Here's how the part is built. I have some questions about the finished solid (model axes, mm). Face numbers are marked on the shaded views. Coordinates: 2 decimals unless noted, no trailing zeros. Write each loop counter-clockwise with the first axis right and the second up, starting at its lowest first coordinate (ties: lowest second). Pieces come first, ordered by that corner, then holes. Notation, with made-up numbers: M -7.5,35 L 31.5,35 A20 cw 31.5,46 Z; hole C 65,51.25 d2. An arc over 180 degrees is marked long. Use a Markdown table: item, result.
```python
from build123d import *

# Parameters (mm, degrees)
CROQUIS1_R              = 5
CROQUIS1_R_2            = 4.05
SALIENTE_EXTRUIR1_DEPTH = 3
CROQUIS5_W              = 3
CROQUIS5_H              = 21
SALIENTE_EXTRUIR3_DEPTH = 8
CROQUIS11_W             = 3
CROQUIS11_H             = 21
SALIENTE_EXTRUIR6_DEPTH = 8
CORTAR_EXTRUIR3_DEPTH   = 34
CORTAR_EXTRUIR4_DEPTH   = 3
SALIENTE_EXTRUIR8_DEPTH = 8
CROQUIS15_R             = 1.55
CORTAR_EXTRUIR6_DEPTH   = 7
CROQUIS16_R             = 2.8
CROQUIS16_R_2           = 1.55
CORTAR_EXTRUIR7_DEPTH   = 3


with BuildPart() as part:
    # Croquis1 → Saliente-Extruir1 (new body)
    with BuildSketch(Plane(origin=(0, 0, 0), x_dir=(1, 0, 0), z_dir=(0, 1, 0))):
        Polygon((0, 32), (25.301087099, 32), (25.301087099, -7), (19.301087099, -13), (-1.698912901, -13), (-7.698912901, -7), (-7.698912901, 32), align=None)
        Circle(CROQUIS1_R, mode=Mode.SUBTRACT)
        with Locations((17, 0)):
            Circle(CROQUIS1_R_2, mode=Mode.SUBTRACT)
    extrude(amount=SALIENTE_EXTRUIR1_DEPTH)

    # Croquis5 → Saliente-Extruir3 (add)
    with BuildSketch(Plane.XZ):
        with Locations((-6.198912901, -18.5)):
            Rectangle(CROQUIS5_W, CROQUIS5_H)
    extrude(amount=SALIENTE_EXTRUIR3_DEPTH)

    # Croquis11 → Saliente-Extruir6 (add)
    with BuildSketch(Plane.XZ):
        with Locations((23.801087099, -18.5)):
            Rectangle(CROQUIS11_W, CROQUIS11_H)
    extrude(amount=SALIENTE_EXTRUIR6_DEPTH)

    # Croquis7 → Cortar-Extruir3 (cut, through all)
    with BuildSketch(Plane.ZY.offset(7.698912901)):
        Polygon((-8, -8), (-12, -8), (-8, -4), align=None)
    extrude(amount=-CORTAR_EXTRUIR3_DEPTH, mode=Mode.SUBTRACT)

    # Croquis9 → Cortar-Extruir4 (cut)
    with BuildSketch(Plane(origin=(0, 3, 0), x_dir=(1, 0, 0), z_dir=(0, 1, 0))):
        Polygon((8.801087099, 10.226497308), (13.801087099, 13.113248654), (13.801087099, 18.886751346), (8.801087099, 21.773502692), (3.801087099, 18.886751346), (3.801087099, 13.113248654), align=None)
    extrude(amount=-CORTAR_EXTRUIR4_DEPTH, mode=Mode.SUBTRACT)

    # Croquis13 → Saliente-Extruir8 (add)
    with BuildSketch(Plane.XZ):
        Polygon((-4.698912901, -29), (-4.698912901, -26), (22.301087099, -26), (22.301087099, -29), (25.301087099, -29), (25.301087099, -32), (-7.698912901, -32), (-7.698912901, -29), align=None)
    extrude(amount=SALIENTE_EXTRUIR8_DEPTH)

    # Croquis15 → Cortar-Extruir6 (cut, through all)
    with BuildSketch(Plane.XY.offset(-26)):
        with Locations((-0.198912901, -4)):
            Circle(CROQUIS15_R)
        with Locations((17.801087099, -4)):
            Circle(CROQUIS15_R)
    extrude(amount=-CORTAR_EXTRUIR6_DEPTH, mode=Mode.SUBTRACT)

    # Croquis16 → Cortar-Extruir7 (cut)
    with BuildSketch(Plane.XY.offset(-26)):
        with Locations((-0.198912901, -4)):
            Circle(CROQUIS16_R)
        with Locations((-0.198912901, -4)):
            Circle(CROQUIS16_R_2, mode=Mode.SUBTRACT)
        with Locations((17.801087099, -4)):
            Circle(CROQUIS16_R)
        with Locations((17.801087099, -4)):
            Circle(CROQUIS16_R_2, mode=Mode.SUBTRACT)
    extrude(amount=-CORTAR_EXTRUIR7_DEPTH, mode=Mode.SUBTRACT)


solid = part.part
```
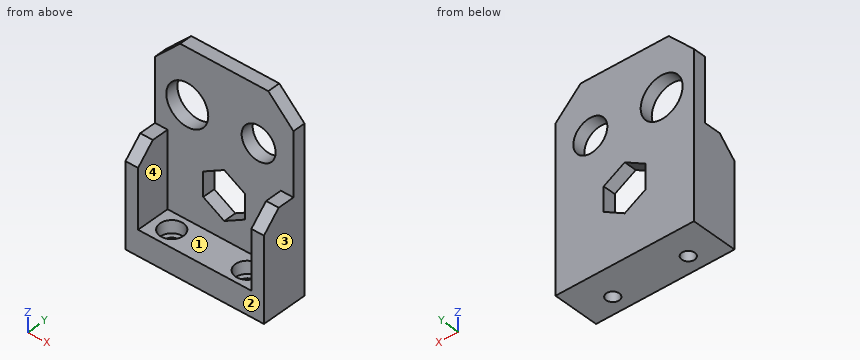
1. Suppose I cut it at C-C on x = 0. Write out the boundary of the cut face in (y, z), and give its area (3 significant figures).
Answers follow:
| item | result |
|---|---|
| outline | M -8,-32 L -5.54,-32 L -5.54,-29 L -6.79,-29 L -6.79,-26 L -8,-26 Z; M -2.46,-32 L 3,-32 L 3,-5 L 0,-5 L 0,-26 L -1.21,-26 L -1.21,-29 L -2.46,-29 Z; M 0,5 L 3,5 L 3,13 L 0,13 Z |
| area | 127 mm2 |
2. I need wall thicknesses on probe 1 along X at (y, z) = (1.65, 0); probe 2 along Z at (x, y) = (4, 2.25); probe 3 along Z at (x, y) = (17, 0.6). Which ranges of each line are inside material? Lowest first, please.
Answers follow:
| item | result |
|---|---|
| probe 1 | x = -7.7 to -5, 5 to 12.95, 21.05 to 25.3 |
| probe 2 | z = -32 to -19, -13 to -3, 3 to 13 |
| probe 3 | z = -32 to -4.05, 4.05 to 13 |
3. Suppose I cut it at A-A on z = 0. Write out the boundary of the cut face in (x, y), and give its area (3 significant figures).
Answers follow:
| item | result |
|---|---|
| outline | M -7.7,0 L -5,0 L -5,3 L -7.7,3 Z; M 5,0 L 12.95,0 L 12.95,3 L 5,3 Z; M 21.05,0 L 25.3,0 L 25.3,3 L 21.05,3 Z |
| area | 44.7 mm2 |
4. Will these pins go through, and if not, where does the flat tip stop? pin 1 Ø3.5 at (x, y) = (17.8, -4) entering from +Z; pin 2 Ø0.9 at (x, y) = (-5.5, -1) entering from +Z; pin 3 Ø9 at (x, z) = (0, 0) entering from +Y; pin 4 Ø12 at (x, z) = (15, 3) entering from -Y.
Answers follow:
| item | result |
|---|---|
| pin 1 | stops at z = -29 |
| pin 2 | stops at z = -8 |
| pin 3 | passes through |
| pin 4 | stops at y = 0 |
5. Suppose I cut it at D-D on z = -24. Write out the boundary of the cut face in (x, y).
Answers follow:
| item | result |
|---|---|
| outline | M -7.7,-8 L -4.7,-8 L -4.7,0 L 22.3,0 L 22.3,-8 L 25.3,-8 L 25.3,3 L -7.7,3 Z |
6. Suppose I cut it at B-B on y = 2. Write out the boundary of the cut face in (x, z), and give its area (3 significant figures).
Answers follow:
| item | result |
|---|---|
| outline | M -7.7,-32 L 25.3,-32 L 25.3,7 L 19.3,13 L -1.7,13 L -7.7,7 Z; hole C 0,0 d10; hole M 3.8,-18.89 L 8.8,-21.77 L 13.8,-18.89 L 13.8,-13.11 L 8.8,-10.23 L 3.8,-13.11 Z; hole C 17,0 d8.1 |
| area | 1,230 mm2 |
7. We'd pull the mould along X, two halves only. Please class the marked faces 1, 2, 3 and 4: +X half, -X half, draft (parallel to the pull), parting line (faces both ways), or undercut.
Answers follow:
| item | result |
|---|---|
| face 1 | undercut |
| face 2 | draft |
| face 3 | +X half |
| face 4 | undercut |
